For this review, take the finished solid that the model builds, in its own axes (mm). Round coordinates to 2 decimals unless told otherwise and drop trailing zeros. Order: outer loops, then holes, each group sorted by start corner. A loop starts at its lowest first (then second) coordinate and runs counter-clockwise, first axis right, second up. Notation, with made-up numbers: (-3, -29) -> (25, -29) arc R23 ccw to (25, -14) -> close; hole circle Ø9 at (25.5, 78.25). An arc over 180 degrees is marked (long way). Answer in a Markdown table with one row per item.
Autodesk Inventor part; units mm, degrees
ref_plane "YZ Plane" through (0, 0, 0) normal (1, 0, 0) x (0, 1, 0)
ref_plane "XZ Plane" through (0, 0, 0) normal (0, 1, 0) x (-1, 0, 0)
ref_plane "XY Plane" through (0, 0, 0) normal (0, 0, 1) x (1, 0, 0)
sketch "Sketch1" plane through (0, 0, 0) normal (0, 0, 1) x (1, 0, 0)
  line L0 (0, 0) -> (406.4, 0)
  line L1 (406.4, 0) -> (406.4, 25.4)
  line L2 (406.4, 25.4) -> (0, 25.4)
  line L3 (0, 25.4) -> (0, 0)
  dimension "d0" = 406.4
  dimension "d1" = 25.4
extrude "Extrusion1" add sketch "Sketch1" along normal blind 6.35
fillet "Fillet1" radius 12.7 1 edges at (406.4, 25.4, 3.175)
fillet "Fillet2" radius 12.7 1 edges at (406.4, 0, 3.175)
fillet "Fillet3" radius 12.7 1 edges at (0, 25.4, 3.175)
fillet "Fillet4" radius 12.7 1 edges at (0, 0, 3.175)
shell "Shell1" thickness 2.54 removed faces 2 at (266.7, 8.4667, 6.35) at (266.7, 8.4667, 0)
properties part number "16inchliftwire"
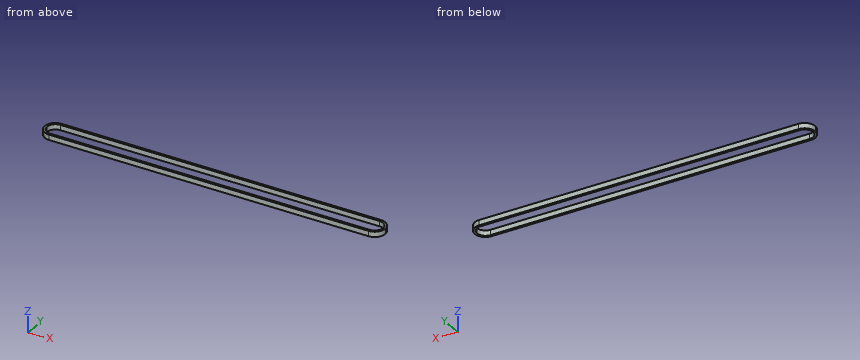
Q1. Clearance check with a flat-ended pin moving along its axis: pin 1 Ø4 at (x, y) = (76, 21) entering from +Z. State where the tip first meets the part, or that it passes through.
Answer key:
| item | result |
|---|---|
| pin 1 | stops at z = 6.35 |
Q2. Take a section at A-A, the plane x = 97. Write out the cut boundary in (y, z), then the cut area to 3 significant figures.
Answer key:
| item | result |
|---|---|
| outline | (0, 0) -> (2.54, 0) -> (2.54, 6.35) -> (0, 6.35) -> close; (22.86, 0) -> (25.4, 0) -> (25.4, 6.35) -> (22.86, 6.35) -> close |
| area | 32.3 mm^2 |
Q3. Take a section at B-B, the plane y = 17. Write out the cut boundary in (x, z), then the cut area to 3 significant figures.
Answer key:
| item | result |
|---|---|
| outline | (0.75, 0) -> (3.49, 0) -> (3.49, 6.35) -> (0.75, 6.35) -> close; (402.91, 0) -> (405.65, 0) -> (405.65, 6.35) -> (402.91, 6.35) -> close |
| area | 34.9 mm^2 |
Q4. To check wall thickness, follow probe 1 along Y at (x, z) = (84.5, 4.25); probe 2 along X at (y, z) = (10, 4); probe 3 along X at (y, z) = (11, 4). State the ranges of each line that lie inside material, in increasing order.
Answer key:
| item | result |
|---|---|
| probe 1 | y = 0 to 2.54, 22.86 to 25.4 |
| probe 2 | x = 0.29 to 2.91, 403.49 to 406.11 |
| probe 3 | x = 0.11 to 2.68, 403.72 to 406.29 |
